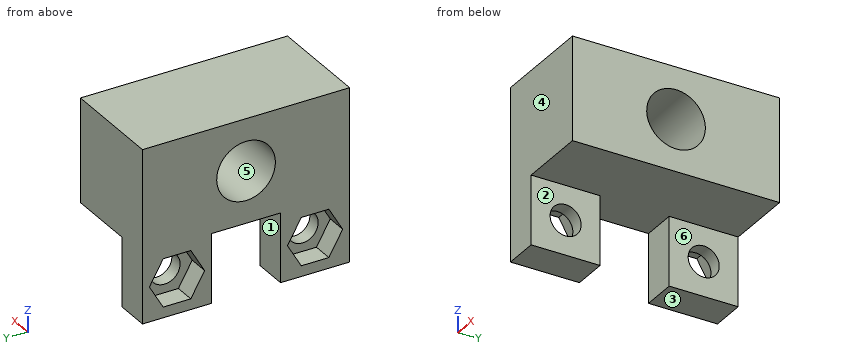
```python
from build123d import *

# Parameters (mm, degrees)
BOSS_EXTRUDE1_DEPTH = 5
SKETCH2_W           = 15
SKETCH2_H           = 30
BOSS_EXTRUDE2_DEPTH = 10
SKETCH3_R           = 4.25
CUT_EXTRUDE1_DEPTH  = 15
SKETCH4_R           = 2.25
CUT_EXTRUDE2_DEPTH  = 15
CUT_EXTRUDE3_DEPTH  = 3


with BuildPart() as part:
    # Sketch1 → Boss-Extrude1 (new body)
    with BuildSketch(Plane(origin=(0, 0, 0), x_dir=(0, 0, -1), z_dir=(1, 0, 0))):
        Polygon((25, 0), (25, 10), (15, 10), (15, 20), (25, 20), (25, 30), (0, 30), (0, 0), align=None)
    extrude(amount=BOSS_EXTRUDE1_DEPTH)

    # Sketch2 → Boss-Extrude2 (add)
    with BuildSketch(Plane(origin=(5, 0, 0), x_dir=(0, 0, -1), z_dir=(1, 0, 0))):
        with Locations((7.5, 15)):
            Rectangle(SKETCH2_W, SKETCH2_H)
    extrude(amount=BOSS_EXTRUDE2_DEPTH)

    # Sketch3 → Cut-Extrude1 (cut)
    with BuildSketch(Plane(origin=(15, 0, 0), x_dir=(0, 0, -1), z_dir=(1, 0, 0))):
        with Locations((7.5, 15)):
            Circle(SKETCH3_R)
    extrude(amount=-CUT_EXTRUDE1_DEPTH, mode=Mode.SUBTRACT)

    # Sketch4 → Cut-Extrude2 (cut)
    with BuildSketch(Plane(origin=(5, 0, 0), x_dir=(0, 0, -1), z_dir=(1, 0, 0))):
        with Locations((20, 25)):
            Circle(SKETCH4_R)
        with Locations((20, 5)):
            Circle(SKETCH4_R)
    extrude(amount=-CUT_EXTRUDE2_DEPTH, mode=Mode.SUBTRACT)

    # Sketch5 → Cut-Extrude3 (cut)
    with BuildSketch(Plane.ZY):
        Polygon((-20, 29), (-23.464101615, 27), (-23.464101615, 23), (-20, 21), (-16.535898385, 23), (-16.535898385, 27), align=None)
        Polygon((-20, 9), (-23.464101615, 7), (-23.464101615, 3), (-20, 1), (-16.535898385, 3), (-16.535898385, 7), align=None)
    extrude(amount=-CUT_EXTRUDE3_DEPTH, mode=Mode.SUBTRACT)


solid = part.part
```
Check sheet for the modelled part. Datum: model origin and axes. Units: mm. Face numbers are marked on the shaded views. A direction names the side the tool comes from. Coordinates: 2 decimals unless noted, no trailing zeros. Write each loop counter-clockwise with the first axis right and the second up, starting at its lowest first coordinate (ties: lowest second). Pieces come first, ordered by that corner, then holes. Notation, with made-up numbers: (-17, 22.5) -> (9, 22.5) arc R13 cw to (9, 39.5) -> close; hole circle Ø3 at (56, 43.5). An arc over 180 degrees is marked (long way). Use a Markdown table: item, result.
1. Sectioned sample at A-A (y = 5). Enter the section's corners in (x, z).
Reported:
| item | result |
|---|---|
| outline | (0, -25) -> (5, -25) -> (5, -22.25) -> (3, -22.25) -> (3, -23.46) -> (0, -23.46) -> close; (0, -16.54) -> (3, -16.54) -> (3, -17.75) -> (5, -17.75) -> (5, -15) -> (15, -15) -> (15, 0) -> (0, 0) -> close |
2. Tool access check on the marked faces 1, 2 and 3. Record the directions out of +Z, -Z, +X, -X, +Y, -Y that give a thin tool (end or side, any length) a straight path to the whole face; none if there is none.
Reported:
| item | result |
|---|---|
| face 1 | -Z, +X, -X |
| face 2 | -Z, +X, +Y, -Y |
| face 3 | -Z, +X, -X, +Y, -Y |
3. Sectioned sample at D-D (z = -7.5). Enter the section's corners in (x, y).
Reported:
| item | result |
|---|---|
| outline | (0, 0) -> (15, 0) -> (15, 10.75) -> (0, 10.75) -> close; (0, 19.25) -> (15, 19.25) -> (15, 30) -> (0, 30) -> close |
4. Sectioned sample at B-B (x = 4.25). Enter the section's corners in (y, z).
Reported:
| item | result |
|---|---|
| outline | (0, -25) -> (10, -25) -> (10, -15) -> (20, -15) -> (20, -25) -> (30, -25) -> (30, 0) -> (0, 0) -> close; hole circle Ø4.5 at (5, -20); hole circle Ø8.5 at (15, -7.5); hole circle Ø4.5 at (25, -20) |
5. Release check for a two-part mould opening along Y. For the marked faces 4, 5 and 6 record: pulls with the +Y half, pulls with the -Y half, needs draft (parallel to the pull), parting line crosses it, or undercut.
Reported:
| item | result |
|---|---|
| face 4 | pulls with the -Y half |
| face 5 | undercut |
| face 6 | needs draft |
6. Go/stop test with flat-tipped pins: pin 1 Ø3.5 at (x, y) = (2, 24) entering from +Z; pin 2 Ø7.5 at (x, y) = (11, 7.5) entering from -Z; pin 3 Ø1.5 at (y, z) = (19.5, -22) entering from +X; pin 4 Ø6 at (y, z) = (5, -20) entering from -X. Record where each tip stops, or that it passes through.
Reported:
| item | result |
|---|---|
| pin 1 | stops at z = 0 |
| pin 2 | stops at z = -15 |
| pin 3 | stops at x = 5 |
| pin 4 | stops at x = 3 |
7. Scan lines: line 1 along Y through (x, z) = (3.45, -20); line 2 along Z through (x, y) = (1.25, 4.5); line 3 along Y through (x, z) = (5.25, -10). Record each from-to range of solid material in increasing order.
Reported:
| item | result |
|---|---|
| line 1 | y = 0 to 2.75, 7.25 to 10, 20 to 22.75, 27.25 to 30 |
| line 2 | z = -25 to -23.46, -16.54 to 0 |
| line 3 | y = 0 to 11.56, 18.44 to 30 |
8. Sectioned sample at C-C (z = -19). Enter the section's corners in (x, y), plus the area to 3 significant figures.
Reported:
| item | result |
|---|---|
| outline | (0, 0) -> (5, 0) -> (5, 2.98) -> (3, 2.98) -> (3, 1.58) -> (0, 1.58) -> close; (0, 8.42) -> (3, 8.42) -> (3, 7.02) -> (5, 7.02) -> (5, 10) -> (0, 10) -> close; (0, 20) -> (5, 20) -> (5, 22.98) -> (3, 22.98) -> (3, 21.58) -> (0, 21.58) -> close; (0, 28.42) -> (3, 28.42) -> (3, 27.02) -> (5, 27.02) -> (5, 30) -> (0, 30) -> close |
| area | 42.8 mm2 |
